Work out the finished part from the listing and answer in its coordinate system (mm). A direction names the side the tool comes from. Coordinates: 2 decimals unless noted, no trailing zeros. Loops run counter-clockwise (first coordinate to the right, second up) from the corner with the lowest first, then second, coordinate; pieces in that order, holes last. Notation, with made-up numbers: (40, 19.25) - (54, 19.25) arc R35 cw to (54, 56.25) - close; hole circle Ø7 at (77, -29). An arc over 180 degrees is marked (long way). Write each question's results on one line, items separated by ' | '. Start each with the question number.
1. Determine the mould class of faces 1 (the cylindrical face through (39.464, 61.59, 0.133)), 2 (the conical face through (84.464, -0.967, 38.133)), 3 (the flat face through (54, -25.4, 45)) for opening direction X: released by +X, released by -X, zero draft, split by the parting line, or undercut.
2. Which of the six approach directions +Z, -Z, +X, -X, +Y, -Y give full straight-line access (tool end or side, diameter ignored) to faces 4 (the flat face through (41.275, -1, 5)), 5 (the flat face through (-3, -7.938, 31)), 6 (the flat face through (22.225, 17, 19)), 7 (the flat face through (54, 25.4, 45))?
3. A cutting plane is placed at B-B on y = 51. Determine the outline of the cut face in (x, z) (3 decimals).
4. Find the intervals of material crossed by line 1 along Z through (x, y) = (0, -47.5) (3 decimals); line 2 along Y through (x, z) = (32, 28); line 3 along Y through (x, z) = (-11.5, 24.5), in increasing order. Write a range as [from, to].
5. Each of these flat-tipped pins is pushed along its axis until it touches: P1, Ø3, axis at y = -6.5, z = 65, coming from the -X side (3 decimals); P2, Ø13, axis at x = 71.5, y = -12, coming from the +Z side; P3, Ø3, axis at x = 93, z = 51.5, coming from the +Y side. Where does it stop, or does it pass through?
6. A cutting plane is placed at A-A on z = -3. Determine the outline of the cut face in (x, y) (3 decimals), then the cut area to 3 significant figures.
from build123d import *

# Parameters (mm, degrees)
F1_DEPTH = 63.5
F2_DEPTH = 25.4
F3_DEPTH = 7.9375
F5_R     = 6.35


with BuildPart() as f1:
    # F0 (on Front) → F1 (new body, symmetric)
    with BuildSketch(Plane.XZ):
        Polygon((22.225, 9.525), (-41.275, 9.525), (-41.275, -9.525), (41.275, -9.525), (41.275, 9.525), align=None)
    extrude(amount=F1_DEPTH, both=True)

    # F0 (on Front) → F2 (join, symmetric)
    with BuildSketch(Plane.XZ):
        with BuildLine():
            Line((22.225, 27.8803942589), (22.225, 9.525))
            Line((22.225, 9.525), (41.275, 9.525))
            Line((41.275, 9.525), (41.275, 27.8803942589))
            ThreePointArc((41.275, 27.8803942589), (45.9246798487, 39.1057144102), (57.15, 43.7553942589))
            Line((57.15, 43.7553942589), (60.325, 43.7553942589))
            Line((60.325, 43.7553942589), (60.325, 62.8053942589))
            Line((60.325, 62.8053942589), (57.15, 62.8053942589))
            add(Edge.make_bspline(
                [(54.9804315881, 62.7379414747), (55.7065758569, 62.765977986), (56.4298660875, 62.7884783704), (57.15, 62.8053942589)],
                knots=[110.0629711844, 110.0629711844, 110.0629711844, 110.0629711844, 111.9208695346, 111.9208695346, 111.9208695346, 111.9208695346], degree=3))
            ThreePointArc((54.9804315881, 62.7379414747), (31.6987937242, 51.7967427282), (22.225, 27.8803942589))
        make_face()
        Polygon((60.325, 66.675), (60.325, 62.8053942589), (60.325, 43.7553942589), (85.7897415942, 43.7553942589), (86.0521197319, 66.675), align=None)
    extrude(amount=F2_DEPTH, both=True)

    # F0 (on Front) → F3 (join, symmetric)
    with BuildSketch(Plane.XZ):
        with BuildLine():
            add(Edge.make_bspline(
                [(-41.275, 9.525), (-41.0700733104, 39.9874044881), (11.9632257601, 61.0770423539), (54.9804315881, 62.7379414747)],
                knots=[0, 0, 0, 0, 110.0629711844, 110.0629711844, 110.0629711844, 110.0629711844], degree=3))
            Line((-41.275, 9.525), (22.225, 9.525))
            Line((22.225, 9.525), (22.225, 27.8803942589))
            ThreePointArc((22.225, 27.8803942589), (31.6987937242, 51.7967427282), (54.9804315881, 62.7379414747))
        make_face()
    extrude(amount=F3_DEPTH, both=True)

    # F0 (on Front) → F4 (revolve)
    with BuildSketch(Plane.XZ):
        Polygon((86.0521197319, 66.675), (85.7897415942, 43.7553942589), (85.725, 38.1), (111.125, 38.1), (111.125, 66.675), align=None)
    revolve(axis=Axis((85.888559866, 0, 52.3875), (0.0114470096, 0, 0.9999344808)))

    # F5
    f5_edges = [f1.edges().sort_by_distance(p)[0] for p in [
        (41.275, -63.5, 0),
        (-41.275, -63.5, 0),
        (-41.275, 63.5, 0),
        (41.275, 63.5, 0),
    ]]
    fillet(f5_edges, radius=F5_R)


solid = f1.part
Values:
1) face 1: released by +X | face 2: undercut | face 3: zero draft
2) face 4: -Z, +X, +Y, -Y | face 5: +Z, -X, -Y | face 6: +Z, -X, +Y | face 7: +Z, +X, -X, +Y
3) outline: (-41.275, -9.525) - (41.275, -9.525) - (41.275, 9.525) - (-41.275, 9.525) - close
4) line 1: [-9.525, 9.525] | line 2: [-25.4, 25.4] | line 3: [-7.94, 7.94]
5) P1: x = 60.325 | P2: z = 67.2 | P3: y = 24.61
6) outline: (-41.275, -57.15) arc R6.35 ccw to (-34.925, -63.5) - (34.925, -63.5) arc R6.35 ccw to (41.275, -57.15) - (41.275, 57.15) arc R6.35 ccw to (34.925, 63.5) - (-34.925, 63.5) arc R6.35 ccw to (-41.275, 57.15) - close | area: 10,400 mm^2
